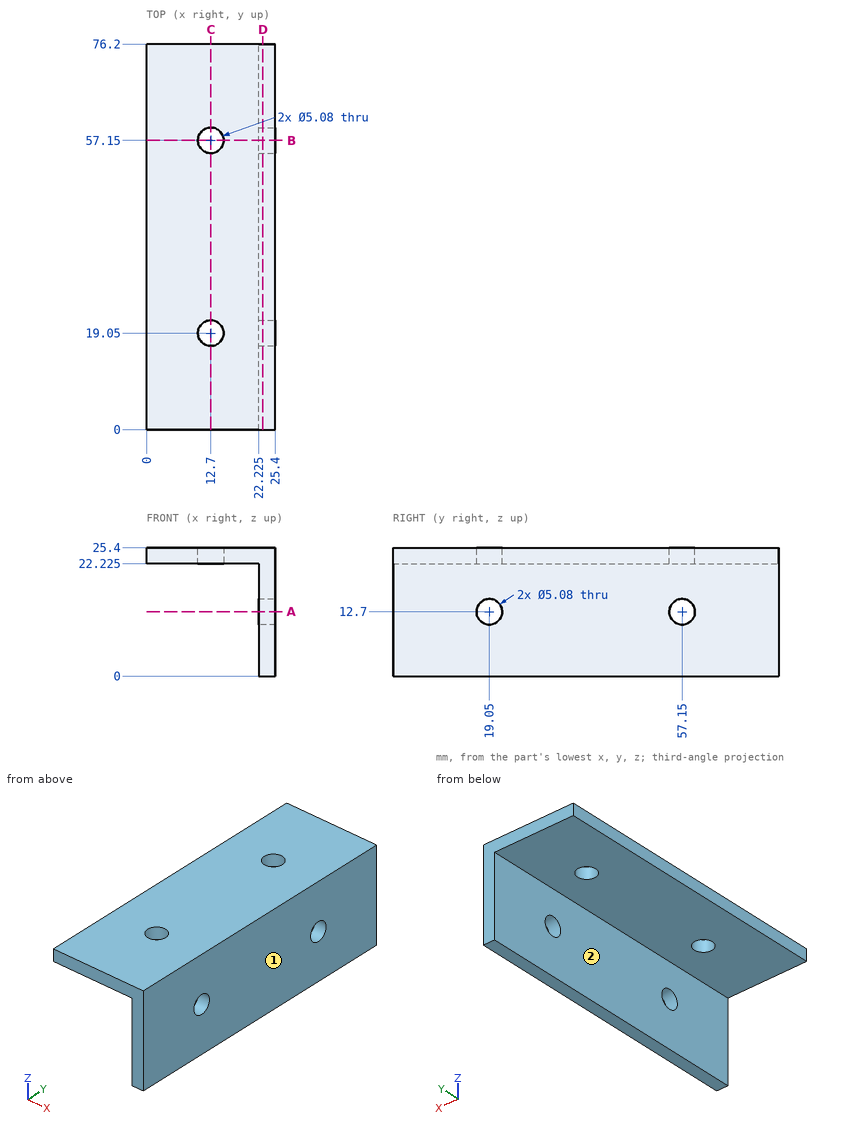
Job drawing, mm, ordinate dimensions from the low corner. One solid piece. A direction names the side the tool comes from. Give positions to 0.01 mm unless a question says otherwise; leave off trailing zeros. Write each loop counter-clockwise with the first axis right and the second up, starting at its lowest first coordinate (ties: lowest second). Pieces come first, ordered by that corner, then holes. Notation, with made-up numbers: M 68.5,88.25 L 91.5,88.25 A17 cw 91.5,119.25 Z; hole C 82.5,59.5 d1. An arc over 180 degrees is marked long. Put each result on its own line as item: value. Start each with the question number.
(1) Band-saw the part on C-C, the plane x = 12.7. Write the cut outline in (y, z) (3 decimals), and give its area (3 significant figures).
(2) Probe L1, parallel to Y at x = 23.2, z = 12.7; L2, parallel to X at y = 19.05, z = 23.45. List the from-to ranges inside material, lowest first.
(3) Flat gauge pins, fed straight in: pin 1 Ø4 at (y, z) = (46, 9.5) entering from -X (3 decimals); pin 2 Ø4 at (x, y) = (12.7, 57.15) entering from +Z. Where does each tip first touch, or does it go through?
(4) Which spindle directions (+Z, -Z, +X, -X, +Y, -Y) get a long thin tool onto all of the face, cutting with end or side? Do the marked faces 1 and 2. Say none if no direction does.
(5) Band-saw the part on B-B, the plane y = 57.15. Write the cut outline in (x, z) (3 decimals), and give its area (3 significant figures).
(6) Band-saw the part on D-D, the plane x = 23. Write the cut outline in (y, z).
(7) Band-saw the part on A-A, the plane z = 12.7. Write the cut outline in (x, y) (3 decimals).
Response values:
1. outline: M 0,22.225 L 16.51,22.225 L 16.51,25.4 L 0,25.4 Z; M 21.59,22.225 L 54.61,22.225 L 54.61,25.4 L 21.59,25.4 Z; M 59.69,22.225 L 76.2,22.225 L 76.2,25.4 L 59.69,25.4 Z
1. area: 210 mm2
2. L1: y = 0 to 16.51, 21.59 to 54.61, 59.69 to 76.2
2. L2: x = 0 to 10.16, 15.24 to 25.4
3. pin 1: stops at x = 22.225
3. pin 2: passes through
4. face 1: +Z, -Z, +X, +Y, -Y
4. face 2: -Z, -X, +Y, -Y
5. outline: M 0,22.225 L 10.16,22.225 L 10.16,25.4 L 0,25.4 Z; M 15.24,22.225 L 22.225,22.225 L 22.225,15.24 L 25.4,15.24 L 25.4,25.4 L 15.24,25.4 Z; M 22.225,0 L 25.4,0 L 25.4,10.16 L 22.225,10.16 Z
5. area: 119 mm2
6. outline: M 0,0 L 76.2,0 L 76.2,25.4 L 0,25.4 Z; hole C 19.05,12.7 d5.08; hole C 57.15,12.7 d5.08
7. outline: M 22.225,0 L 25.4,0 L 25.4,16.51 L 22.225,16.51 Z; M 22.225,21.59 L 25.4,21.59 L 25.4,54.61 L 22.225,54.61 Z; M 22.225,59.69 L 25.4,59.69 L 25.4,76.2 L 22.225,76.2 Z
